Could you check a few things on this model? Use its own coordinates, in mm. Face numbers are marked on the shaded views. A direction names the side the tool comes from. Round coordinates to 2 decimals unless told otherwise and drop trailing zeros. Loops run counter-clockwise (first coordinate to the right, second up) from the corner with the lowest first, then second, coordinate; pieces in that order, holes last. Notation, with made-up numbers: (85, 84) - (117, 84) arc R25 ccw to (117, 100) - close; hole circle Ø6 at (26, 14). An arc over 180 degrees is marked (long way). Use one line per item in the form item = value.
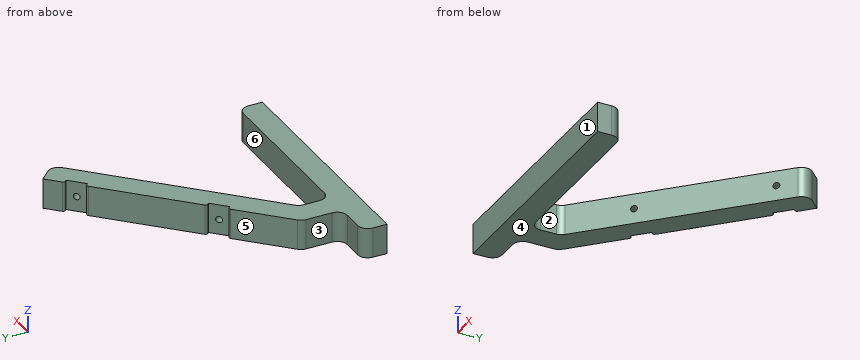
```python
from build123d import *

# Parameters (mm, degrees)
F1_DEPTH = 15
F2_R     = 5
F3_W     = 10
F3_H     = 15
F4_DEPTH = 2
F5_D     = 3.2
F5_DEPTH = 25
F5_TIP   = 0.9613769904
F6_R     = 1


with BuildPart() as f1:
    # F0 (on Top) → F1 (new body)
    with BuildSketch(Plane.XY):
        Polygon((-40, 6), (-28, 6), (-28, 21.0294372515), (53.3380951166, 102.3675323681), (44.8528137424, 110.8528137424), (-40, 26), align=None)
        Polygon((-60, -6), (60, -6), (60, 6), (-28, 6), (-40, 6), (-60, 6), align=None)
    extrude(amount=F1_DEPTH)

    # F2
    f2_edges = [f1.edges().sort_by_distance(p)[0] for p in [
        (-40, 6, 7.5),
        (-28, 6, 7.5),
        (-60, 6, 7.5),
        (60, 6, 7.5),
        (53.338095, 102.367532, 7.5),
        (-40, 26, 7.5),
        (-28, 21.029437, 7.5),
    ]]
    fillet(f2_edges, radius=F2_R)

    # F3 (on face) → F4 (cut)
    with BuildSketch(Plane(origin=(-33, 33, 0), x_dir=(-0.7071067812, -0.7071067812, 0), z_dir=(-0.7071067812, 0.7071067812, 0))):
        with Locations((-95.1005050634, 7.5)):
            Rectangle(F3_W, F3_H)
        with Locations((-29.1005050634, 7.5)):
            Rectangle(F3_W, F3_H)
    extrude(amount=-F4_DEPTH, mode=Mode.SUBTRACT)

    # F5
    with Locations(Plane(origin=(-33, 33, 0), x_dir=(-0.7071067812, -0.7071067812, 0), z_dir=(-0.7071067812, 0.7071067812, 0))):
        with Locations((-95.1005050634, 7.5), (-29.1005050634, 7.5)):
            Hole(F5_D / 2, depth=F5_DEPTH)
            with Locations((0, 0, -(F5_DEPTH + F5_TIP / 2))):  # 118° drill point
                Cone(0, F5_D / 2, F5_TIP, mode=Mode.SUBTRACT)

    # F6
    f6_edges = [f1.edges().sort_by_distance(p)[0] for p in [
        (37.781746, 103.781746, 7.5),
        (30.710678, 96.710678, 7.5),
        (-8.887302, 57.112698, 7.5),
        (-15.958369, 50.041631, 7.5),
    ]]
    fillet(f6_edges, radius=F6_R)


solid = f1.part
```
1. If we section it at C-C, the plane x = 41.5: Count the separate pieces of the cut face and the enclosed holes in it, plus the area to 3 significant figures.
Solution:
separate_pieces = 2
enclosed_holes = 1
area = 423 mm^2
2. If we section it at B-B, the plane x = -50: Write out the boundary of the cut face in (y, z).
Solution:
outline = (-6, 0) - (6, 0) - (6, 15) - (-6, 15) - close
3. We'd pull the mould along Y, two halves only. Please class the marked faces 4, 5 and 6: +Y half, -Y half, draft (parallel to the pull), parting line (faces both ways), or undercut.
Solution:
face_4 = draft
face_5 = +Y half
face_6 = undercut
4. On a 3-axis mill with a long thin cutter (end or side, diameter ignored), from which of +Z, -Z, +X, -X, +Y, -Y can I reach the whole of each face in a straight line? I mean the marked faces 1, 2 and 3. Say none if no direction works.
Solution:
face_1 = +Z, -Z, +X, -X, -Y
face_2 = +Z, -Z, +X
face_3 = +Z, -Z, -X, +Y
5. Please list where these lines run through material, in increasing order: line 1 along Y through (x, z) = (37, 8.25); line 2 along X through (y, z) = (10.5, 1.5); line 3 along Y through (x, z) = (-16, 12.25).
Solution:
line_1 = -6 to 6, 86.03 to 95.49, 99.49 to 100.17
line_2 = -40.03 to -27.97
line_3 = -6 to 6, 33.03 to 49.63
6. For P1, Ø6, axis at x = -35.5, z = 12, coming from the +Y side; P2, Ø5, axis at y = 50, z = 2.5, coming from the -X side; P3, Ø3, axis at x = 11.5, z = 2, coming from the +Y side, each with a flat end and sliding along its axis, tell me the tip position at first contact or that it passes through.
Solution:
P1 = 33.5
P2 = -18.5
P3 = 79
7. If we section it at D-D, the plane y = 59.5: Write out the boundary of the cut face in (x, z), plus the area to 3 significant figures.
Solution:
outline = (-6.5, 0) - (10.47, 0) - (10.47, 15) - (-6.5, 15) - close
area = 255 mm^2
